For this review, use the dimensioned drawing (mm, ordinates from the lowest corner) and the shaded views. A direction names the side the tool comes from. Give positions to 0.01 mm unless a question says otherwise; leave off trailing zeros. Loops run counter-clockwise (first coordinate to the right, second up) from the corner with the lowest first, then second, coordinate; pieces in that order, holes last. Notation, with made-up numbers: M 15.5,70 L 44.5,70 A34 cw 44.5,102 Z; hole C 23,-11.5 d1. An arc over 180 degrees is marked long. Return JSON: item names as keys, results as strings.
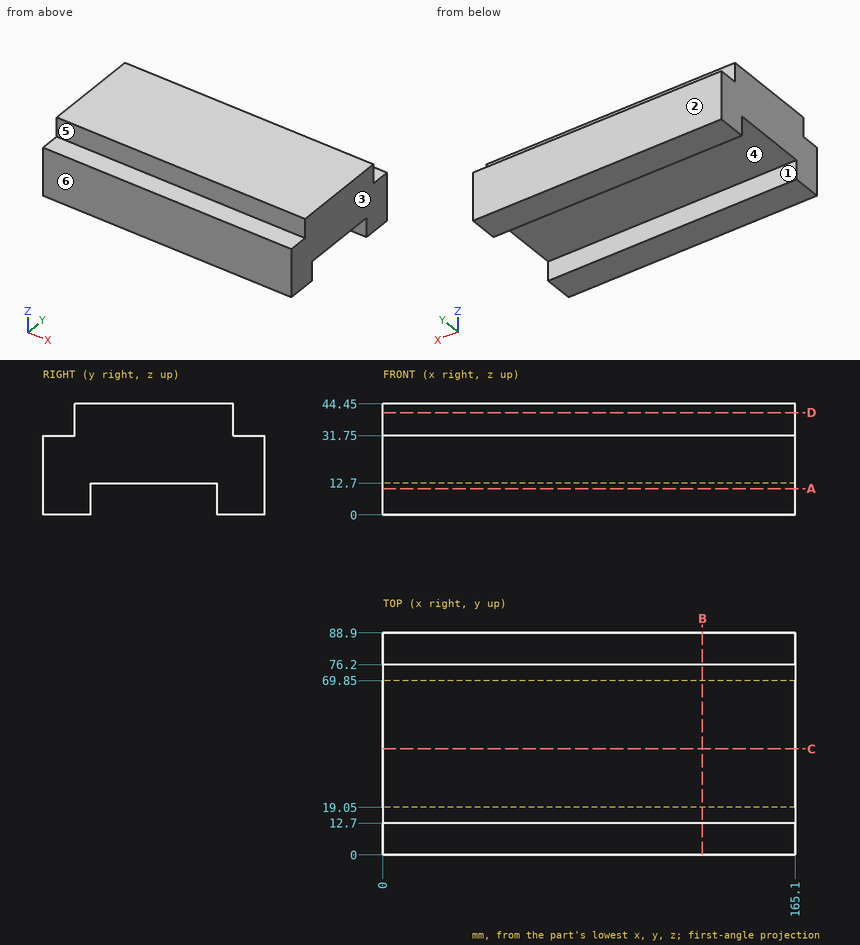
1) Consider section B-B on x = 128. Write out the cut boundary in (y, z).
From the geometry:
{"outline": "M 0,0 L 19.05,0 L 19.05,12.7 L 69.85,12.7 L 69.85,0 L 88.9,0 L 88.9,31.75 L 76.2,31.75 L 76.2,44.45 L 12.7,44.45 L 12.7,31.75 L 0,31.75 Z"}
2) Consider section D-D on z = 41. Write out the cut boundary in (x, y).
From the geometry:
{"outline": "M 0,12.7 L 165.1,12.7 L 165.1,76.2 L 0,76.2 Z"}
3) The part is to be moulded in two halves that separate along Y. For the marked faces 1, 2 and 3, say which applies: released by +Y, released by -Y, zero draft, split by the parting line, or undercut.
From the geometry:
{"face 1": "undercut", "face 2": "released by +Y", "face 3": "zero draft"}
4) Consider section A-A on z = 10.5. Write out the cut boundary in (x, y), then the cut area to 3 significant figures.
From the geometry:
{"outline": "M 0,0 L 165.1,0 L 165.1,19.05 L 0,19.05 Z; M 0,69.85 L 165.1,69.85 L 165.1,88.9 L 0,88.9 Z", "area": "6,290 mm²"}
5) Insertion check: pin 1 (10 mm diameter, centred on x = 113, z = 38.5, fed in from -Y); pin 2 (10 mm diameter, centred on x = 106, y = 85.5, fed in from +Z); pin 3 (10 mm diameter, centred on x = 70.5, z = 37, fed in from +Y). Each pin has a flat end and moves straight along its axis. Give the tip position at first contact, or say it passes through.
From the geometry:
{"pin 1": "y = 12.7", "pin 2": "z = 31.75", "pin 3": "y = 76.2"}
6) Consider section C-C on y = 42.5. Write out the cut boundary in (x, z), then the cut area to 3 significant figures.
From the geometry:
{"outline": "M 0,12.7 L 165.1,12.7 L 165.1,44.45 L 0,44.45 Z", "area": "5,240 mm²"}
7) Wall thickness on L1, parallel to Y at x = 134, z = 6; L2, parallel to Z at x = 72, y = 45; L3, parallel to Y at x = 9, z = 34: over which ranges is each line inside the solid? List them lowest first. Write a range as from..to.
From the geometry:
{"L1": "0..19.05, 69.85..88.9", "L2": "12.7..44.45", "L3": "12.7..76.2"}
8) Tool access review of the marked faces 4, 5 and 6: name each direction out of +Z, -Z, +X, -X, +Y, -Y from which nothing blocks a thin tool from reaching the whole face with its end or side.
From the geometry:
{"face 4": "-Z, +X, -X", "face 5": "+Z, +X, -X, -Y", "face 6": "+Z, -Z, +X, -X, -Y"}
